Here's how the part is built. I have some questions about the finished solid (model axes, mm). A direction names the side the tool comes from. Round coordinates to 2 decimals unless told otherwise and drop trailing zeros. Loops run counter-clockwise (first coordinate to the right, second up) from the corner with the lowest first, then second, coordinate; pieces in that order, holes last. Notation, with made-up numbers: M 3,80 L 34,80 A8 cw 34,89 Z; hole C -13.75,-1.5 d6. An arc over 180 degrees is marked long. Answer as a JSON object with one key per item and string values.
from build123d import *

# Parameters (mm, degrees)
EXTRUDE_1_DEPTH      = 20
EXTRUDE_1_DEPTH_BACK = 20
SKETCH_2_R           = 3.25
CUT_EXTRUDE_1_DEPTH  = 40
FILLET_1_R           = 10


with BuildPart() as part:
    # Sketch 1 → Extrude 1 (new, two sides: drawn at the far end of the back side and taken through both)
    with BuildSketch(Plane.XY.offset(-EXTRUDE_1_DEPTH_BACK)):
        Polygon((-20, 0), (0, 0), (0, -30), (-3, -30), (-3, -3), (-20, -3), align=None)
    extrude(amount=EXTRUDE_1_DEPTH + EXTRUDE_1_DEPTH_BACK)

    # Sketch 2 → Cut-Extrude 1 (cut)
    with BuildSketch(Plane(origin=(0, 0, 0), x_dir=(1, 0, 0), z_dir=(0, 1, 0))):
        with Locations(Location((-10, 0, 0), (0, 0, 270))):
            Circle(SKETCH_2_R)
    extrude(amount=-CUT_EXTRUDE_1_DEPTH, mode=Mode.SUBTRACT)

    # Fillet 1
    fillet_1_edges = [part.edges().sort_by_distance(p)[0] for p in [
        (-20, -1.5, 20),
        (-20, -1.5, -20),
    ]]
    fillet(fillet_1_edges, radius=FILLET_1_R)


solid = part.part
Item 1: For P1, Ø3, axis at x = -10.5, z = 5, coming from the -Y side, with a flat end and sliding along its axis, tell me the tip position at first contact or that it passes through.
Solution:
{"P1": "stops at y = -3"}
Item 2: I want a section at D-D on y = -6.25. List the corners of the cut face in (x, z) for me, plus the area to 3 significant figures.
Solution:
{"outline": "M -3,-20 L 0,-20 L 0,20 L -3,20 Z", "area": "120 mm2"}
Item 3: I want a section at A-A on z = 0. List the corners of the cut face in (x, y) for me, plus the area to 4 significant figures.
Solution:
{"outline": "M -20,-3 L -13.25,-3 L -13.25,0 L -20,0 Z; M -6.75,-3 L -3,-3 L -3,-30 L 0,-30 L 0,0 L -6.75,0 Z", "area": "121.5 mm2"}
Item 4: I want a section at C-C on z = 7. List the corners of the cut face in (x, y) for me.
Solution:
{"outline": "M -20,-3 L -3,-3 L -3,-30 L 0,-30 L 0,0 L -20,0 Z"}
Item 5: I want a section at B-B on x = -7.25. List the corners of the cut face in (y, z) for me, plus the area to 3 significant figures.
Solution:
{"outline": "M -3,-20 L 0,-20 L 0,-1.73 L -3,-1.73 Z; M -3,1.73 L 0,1.73 L 0,20 L -3,20 Z", "area": "110 mm2"}
Item 6: For faces 1 (the face through (-3, -17, 0)), 2 (the face through (0, -15, 0)), which set-ups out of +Z, -Z, +X, -X, +Y, -Y let a thin tool reach every point of the face, with its end or its side?
Solution:
{"face 1": "+Z, -Z, -X, -Y", "face 2": "+Z, -Z, +X, +Y, -Y"}
Item 7: If I drill on L1, parallel to X at y = -1.5, z = 0; L2, parallel to X at y = -4, z = -13.5, over which ranges is the centre line in solid material (lowest first)? Write a range as from..to.
Solution:
{"L1": "x = -20..-13.25, -6.75..0", "L2": "x = -3..0"}
